Geometry check sheet. Reference: the model listing, model coordinates, mm. A direction names the side the tool comes from. Give positions to 0.01 mm unless a question says otherwise; leave off trailing zeros. Write each loop counter-clockwise with the first axis right and the second up, starting at its lowest first coordinate (ties: lowest second). Pieces come first, ordered by that corner, then holes. Notation, with made-up numbers: (63, 11) -> (85, 11) arc R15 ccw to (85, 35) -> close; hole circle Ø3 at (36.5, -19.75). An arc over 180 degrees is marked (long way). One line per item, written item: value.
from build123d import *

# Parameters (mm, degrees)
F0_R     = 11.05
F0_R_2   = 9.4
F1_DEPTH = 3.5
F0_R_3   = 5.75
F0_R_4   = 4
F2_DEPTH = 2.5
F3_SIZE  = 0.4


with BuildPart() as f1:
    # F0 (on Top) → F1 (new body, symmetric)
    with BuildSketch(Plane.XY):
        Circle(F0_R)
        Circle(F0_R_2, mode=Mode.SUBTRACT)
    extrude(amount=F1_DEPTH, both=True)



with BuildPart() as f1b:
    # F0 (on Top) → F1, piece 2 (new body, symmetric)
    with BuildSketch(Plane.XY):
        Circle(F0_R_3)
        Circle(F0_R_4, mode=Mode.SUBTRACT)
    extrude(amount=F1_DEPTH, both=True)


with BuildPart() as f1_1:
    add(f1.part)

    add(f1b.part)  # F2 merges F1b
    # F0 (on Top) → F2 (join, symmetric)
    with BuildSketch(Plane.XY):
        Circle(F0_R_2)
        Circle(F0_R_3, mode=Mode.SUBTRACT)
    extrude(amount=F2_DEPTH, both=True)

    # F3
    f3_edges = [f1_1.edges().sort_by_distance(p)[0] for p in [
        (-11.05, 0, 3.5),
        (-11.05, 0, -3.5),
        (-4, 0, 3.5),
        (-5.75, 0, 3.5),
        (-5.75, 0, -3.5),
        (-4, 0, -3.5),
    ]]
    chamfer(f3_edges, length=F3_SIZE)


solid = f1_1.part
1) Depth check by flat-ended pin: pin 1 Ø3 at (x, z) = (-7, 2.5) entering from +Y; pin 2 Ø4 at (x, z) = (-3, 1.5) entering from +Y; pin 3 Ø7 at (x, y) = (0, 0) entering from -Z. Enter the tip coordinate at first touch or a pass-through.
Verdict:
pin 1: y = 9.58
pin 2: y = 11
pin 3: through
2) Mould release check, pull along X, two halves, no side actions. Record for faces 1 (the cylindrical face through (-2.038, -9.176, 2.993)), 2 (the flat face through (-3, -4, -3.5)), 3 (the cylindrical face through (-2.395, -10.787, 0.043)): released by +X, released by -X, zero draft, split by the parting line, or undercut.
Verdict:
face 1: undercut
face 2: zero draft
face 3: split by the parting line
3) Tool access check on faces 4 (the flat face through (-4.31, -4.05, -2.5)), 5 (the cylindrical face through (-0.75, 5.7, 2.8)), 6 (the flat face through (4, -9, -3.5)). Record the directions out of +Z, -Z, +X, -X, +Y, -Y that give a thin tool (end or side, any length) a straight path to the whole face; none if there is none.
Verdict:
face 4: -Z
face 5: +Z
face 6: -Z, +X, -X, +Y, -Y
4) Scan lines: probe 1 along Y at (x, z) = (0, 2.7); probe 2 along Y at (x, z) = (0, 1.25); probe 3 along X at (y, z) = (-1, -2.75). Record each from-to range of solid material in increasing order.
Verdict:
probe 1: -11.05 to -9.4, -5.75 to -4, 4 to 5.75, 9.4 to 11.05
probe 2: -11.05 to -4, 4 to 11.05
probe 3: -11 to -9.35, -5.66 to -3.87, 3.87 to 5.66, 9.35 to 11
5) Sectioned sample at A-A on z = -1.25. Record the cut outline in (x, y), plus the area to 3 significant figures.
Verdict:
outline: circle Ø22.1 at (0, 0); hole circle Ø8 at (0, 0)
area: 333 mm^2
